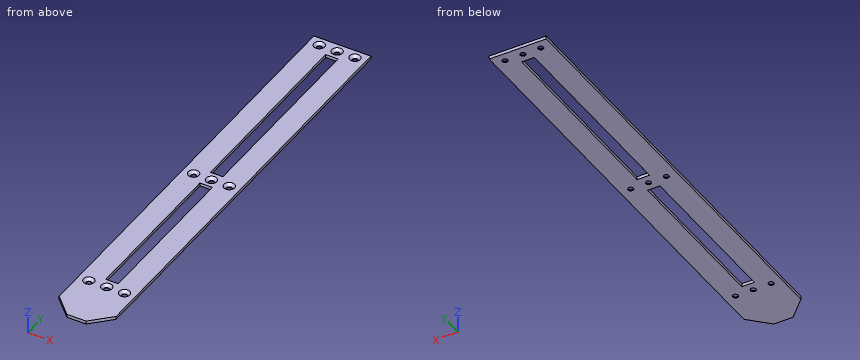
from build123d import *

# Parameters (mm, degrees)
BASE_FLANGE1_START       = -1.755
BASE_FLANGE1_OUTLINE_W   = 14
BASE_FLANGE1_OUTLINE_H   = 180
BASE_FLANGE1_OUTLINE_H_2 = 220
BASE_FLANGE1_DEPTH       = 3.51
SKETCH2_R                = 3
CUT_EXTRUDE2_DEPTH       = 10
CHAMFER1_SIZE            = 3


# Read off the part's stored shape, not the designer's step: Base-Flange1
with BuildPart() as part:
    # Base-Flange1 outline → Base-Flange1 (new body)
    with BuildSketch(Plane.XY.offset(BASE_FLANGE1_START)):
        Polygon((10.786796564, -44.407529677), (32, -23.194326241), (32, 463.194326241), (-32, 463.194326241), (-32, -23.194326241), (-10.786796564, -44.407529677), align=None)
        with Locations((0, 113.194326241)):
            Rectangle(BASE_FLANGE1_OUTLINE_W, BASE_FLANGE1_OUTLINE_H, mode=Mode.SUBTRACT)
        with Locations((0, 333.194326241)):
            Rectangle(BASE_FLANGE1_OUTLINE_W, BASE_FLANGE1_OUTLINE_H_2, mode=Mode.SUBTRACT)
    extrude(amount=BASE_FLANGE1_DEPTH)

    # Sketch2 → Cut-Extrude2 (cut)
    with BuildSketch(Plane.XY.offset(1.755)):
        with Locations((-20, 213.194326241)):
            Circle(SKETCH2_R)
        with Locations((0, 213.194326241)):
            Circle(SKETCH2_R)
        with Locations((20, 213.194326241)):
            Circle(SKETCH2_R)
        with Locations((0, 453.194326241)):
            Circle(SKETCH2_R)
        with Locations((20, 453.194326241)):
            Circle(SKETCH2_R)
        with Locations((-20, 453.194326241)):
            Circle(SKETCH2_R)
        with Locations((0, 13.194326241)):
            Circle(SKETCH2_R)
        with Locations((20, 13.194326241)):
            Circle(SKETCH2_R)
        with Locations((-20, 13.194326241)):
            Circle(SKETCH2_R)
    extrude(amount=-CUT_EXTRUDE2_DEPTH, mode=Mode.SUBTRACT)

    # Chamfer1
    chamfer1_edges = [part.edges().sort_by_distance(p)[0] for p in [
        (-3, 453.194326241, 1.755),
        (17, 453.194326241, 1.755),
        (-23, 13.194326241, 1.755),
        (17, 13.194326241, 1.755),
        (-3, 13.194326241, 1.755),
        (-23, 453.194326241, 1.755),
        (-23, 213.194326241, 1.755),
        (-3, 213.194326241, 1.755),
        (17, 213.194326241, 1.755),
    ]]
    chamfer(chamfer1_edges, length=CHAMFER1_SIZE)


solid = part.part
Here's how the part is built. I have some questions about the finished solid (model axes, mm). Round coordinates to 2 decimals unless told otherwise and drop trailing zeros. Write each loop counter-clockwise with the first axis right and the second up, starting at its lowest first coordinate (ties: lowest second). Pieces come first, ordered by that corner, then holes. Notation, with made-up numbers: (4, -11) -> (15, -11) arc R30 cw to (15, 20) -> close; hole circle Ø3 at (21, -32.5). An arc over 180 degrees is marked (long way). One line per item, written item: value.
1) If I drill on line 1 (Y direction, x = 5, z = 0.2); line 2 (X direction, y = 233.5, z = -0.5); line 3 (Y direction, x = 20, z = -1.4), over which ranges is the centre line in solid material (lowest first)? Write a range as [from, to].
Filled sheet:
line 1: y = [-44.41, 23.19], [203.19, 223.19], [443.19, 463.19]
line 2: x = [-32, -7], [7, 32]
line 3: y = [-35.19, 10.19], [16.19, 210.19], [216.19, 450.19], [456.19, 463.19]
2) Suppose I cut it at A-A on y = 63. List the corners of the cut face in (x, z) for me (3 decimals).
Filled sheet:
outline: (-32, -1.755) -> (-7, -1.755) -> (-7, 1.755) -> (-32, 1.755) -> close; (7, -1.755) -> (32, -1.755) -> (32, 1.755) -> (7, 1.755) -> close
3) Suppose I cut it at B-B on z = -0.15. Give the number of separate pieces and of enclosed holes in the cut face, plus the area to 3 significant figures.
Filled sheet:
separate pieces: 1
enclosed holes: 11
area: 26,000 mm2
4) I'm going to push flat-ended pins straight in: pin 1 Ø5 at (x, y) = (0, 453.19) entering from +Z; pin 2 Ø8 at (x, y) = (20, 453.19) entering from +Z; pin 3 Ø9.5 at (x, y) = (-20, 13.19) entering from +Z. Where does each tip first touch, or does it pass through?
Filled sheet:
pin 1: passes through
pin 2: stops at z = -0.24
pin 3: stops at z = 0.51
